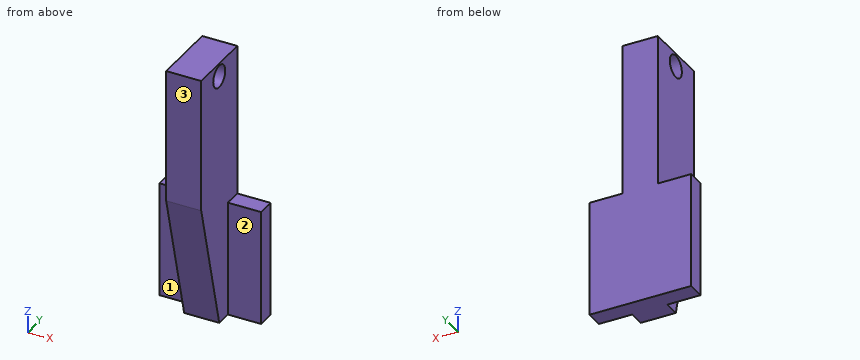
```python
from build123d import *

# Parameters (mm, degrees)
BOSS_EXTRUDE1_DEPTH = 20
SKETCH3_W           = 66
SKETCH3_H           = 10
BOSS_EXTRUDE2_DEPTH = 19.05
SKETCH4_W           = 66
SKETCH4_H           = 10
BOSS_EXTRUDE3_DEPTH = 19.05
SKETCH5_R           = 6.35
CUT_EXTRUDE2_DEPTH  = 40.05


with BuildPart() as part:
    # Sketch1 → Boss-Extrude1 (new body)
    with BuildSketch(Plane(origin=(0, 0, 0), x_dir=(0, 0, -1), z_dir=(1, 0, 0))):
        Polygon((0, -19.05), (76.5, 0), (76.5, 19.05), (-76.5, 19.05), (-76.5, -19.05), align=None)
    extrude(amount=BOSS_EXTRUDE1_DEPTH)

    # Sketch3 → Boss-Extrude2 (add)
    with BuildSketch(Plane(origin=(20, 0, 0), x_dir=(0, 0, -1), z_dir=(1, 0, 0))):
        with Locations((43.5, 14.05)):
            Rectangle(SKETCH3_W, SKETCH3_H)
    extrude(amount=BOSS_EXTRUDE2_DEPTH)

    # Sketch4 → Boss-Extrude3 (add)
    with BuildSketch(Plane.ZY):
        with Locations((-43.5, 14.05)):
            Rectangle(SKETCH4_W, SKETCH4_H)
    extrude(amount=BOSS_EXTRUDE3_DEPTH)

    # Sketch5 → Cut-Extrude2 (cut, through all)
    with BuildSketch(Plane(origin=(20, 0, 0), x_dir=(0, 0, -1), z_dir=(1, 0, 0))):
        with Locations((-68.88, 0)):
            Circle(SKETCH5_R)
    extrude(amount=-CUT_EXTRUDE2_DEPTH, mode=Mode.SUBTRACT)


solid = part.part
```
Geometry check sheet. Reference: the model listing, model coordinates, mm. Face numbers are marked on the shaded views. A direction names the side the tool comes from. Give positions to 0.01 mm unless a question says otherwise; leave off trailing zeros. Loops run counter-clockwise (first coordinate to the right, second up) from the corner with the lowest first, then second, coordinate; pieces in that order, holes last. Notation, with made-up numbers: M -7,34.5 L 19,34.5 A28 ccw 19,65.5 Z; hole C 64,18 d8. An arc over 180 degrees is marked long. Write item = value, one per line. Start each with the question number.
1. Section check A-A, the plane z = 68.88. Enter the section's corners in (x, y), plus the area to 3 significant figures.
2. Section check C-C, the plane x = 4.5. Enter the section's corners in (y, z), plus the area to 3 significant figures.
3. Section check B-B, the plane y = -2. Enter the section's corners in (x, z).
4. Tool access check on the marked faces 1, 2 and 3. Record the directions out of +Z, -Z, +X, -X, +Y, -Y that give a thin tool (end or side, any length) a straight path to the whole face; none if there is none.
5. Go/stop test with flat-tipped pins: P1, Ø5, axis at x = 28.5, y = 14, coming from the +Z side; P2, Ø2, axis at x = -2.5, y = -13, coming from the -Z side; P3, Ø1, axis at y = -1, z = 5, coming from the +X side; P4, Ø9.5, axis at x = -11.5, z = -36, coming from the -Y side. Record where each tip stops, or that it passes through.
6. Thickness scan on probe 1 along Y at (x, z) = (5.25, 68.88); probe 2 along X at (y, z) = (5.5, 34.5); probe 3 along Y at (x, z) = (29, -39). Record the ranges inside material, lowest first.
7. Section check D-D, the plane y = 14. Enter the section's corners in (x, z).
Values follow:
q1.outline = M 0,-19.05 L 20,-19.05 L 20,-6.35 L 0,-6.35 Z; M 0,6.35 L 20,6.35 L 20,19.05 L 0,19.05 Z
q1.area = 508 mm^2
q2.outline = M -19.05,0 L 0,-76.5 L 19.05,-76.5 L 19.05,76.5 L -19.05,76.5 Z; hole C 0,68.88 d12.7
q2.area = 4,970 mm^2
q3.outline = M 0,-68.47 L 20,-68.47 L 20,62.85 L 0,62.85 Z; M 0,74.91 L 20,74.91 L 20,76.5 L 0,76.5 Z
q4.face_1 = +Z, -Z, -X, -Y
q4.face_2 = +Z, -Z, +X, -Y
q4.face_3 = +Z, -Z, +X, -X, -Y
q5.P1 = -10.5
q5.P2 = through
q5.P3 = 20
q5.P4 = 9.05
q6.probe_1 = -19.05 to -6.35, 6.35 to 19.05
q6.probe_2 = 0 to 20
q6.probe_3 = 9.05 to 19.05
q7.outline = M -19.05,-76.5 L 39.05,-76.5 L 39.05,-10.5 L 20,-10.5 L 20,76.5 L 0,76.5 L 0,-10.5 L -19.05,-10.5 Z
